```python
from build123d import *

# Parameters (mm, degrees)
SKETCH1_W           = 27
SKETCH1_H           = 24
BOSS_EXTRUDE1_DEPTH = 37
SHELL1_T            = -3.5
SKETCH3_R           = 2.1
CUT_EXTRUDE1_DEPTH  = 48.349762407
SKETCH5_W           = 74
SKETCH5_H           = 0.5
CUT_EXTRUDE3_DEPTH  = 48.349762407
SWEEP1_START        = -13.5
SWEEP1_DEPTH        = 27
SWEEP1_2_DEPTH      = 3.5
SWEEP1_START_2      = 10
SWEEP1_3_DEPTH      = 3.5


# Read off the part's stored shape, not the designer's step: Sweep1
with BuildPart() as part:
    # Sketch1 → Boss-Extrude1 (new, symmetric)
    with BuildSketch(Plane.XY):
        Rectangle(SKETCH1_W, SKETCH1_H)
    extrude(amount=BOSS_EXTRUDE1_DEPTH, both=True)

    # Shell1
    shell1_openings = [part.faces().sort_by_distance(p)[0] for p in [
        (0, 0, 37),
        (0, 0, -37),
        (0, -12, 0),
    ]]
    offset(amount=SHELL1_T, openings=shell1_openings, kind=Kind.INTERSECTION)

    # Sketch3 → Cut-Extrude1 (cut, through all)
    with BuildSketch(Plane.ZY.offset(13.5)):
        with Locations((-30, -1.5)):
            Circle(SKETCH3_R)
        with Locations((-10, -1.5)):
            Circle(SKETCH3_R)
        with Locations((10, -1.5)):
            Circle(SKETCH3_R)
        with Locations((30, -1.5)):
            Circle(SKETCH3_R)
    extrude(amount=-CUT_EXTRUDE1_DEPTH, mode=Mode.SUBTRACT)

    # Sketch5 → Cut-Extrude3 (cut, through all)
    with BuildSketch(Plane.ZY.offset(13.5)):
        with Locations((0, -11.75)):
            Rectangle(SKETCH5_W, SKETCH5_H)
    extrude(amount=-CUT_EXTRUDE3_DEPTH, mode=Mode.SUBTRACT)

    # Sweep1 outline → Sweep1 (add)
    with BuildSketch(Plane.YZ.offset(SWEEP1_START)):
        with BuildLine():
            Line((14.288034431, 44.256718109), (59.173181861, 108.359351944))
            Line((59.173181861, 108.359351944), (56.306149706, 110.366869471))
            Line((56.306149706, 110.366869471), (11.421002276, 46.264235636))
            ThreePointArc((11.421002276, 46.264235636), (9.247550016, 41.856910443), (8.5, 37))
            Line((8.5, 37), (12, 37))
            ThreePointArc((12, 37), (12.585559344, 40.804440145), (14.288034431, 44.256718109))
        make_face()
    extrude(amount=SWEEP1_DEPTH)

    # Sweep1 2 outline → Sweep1 2 (add)
    with BuildSketch(Plane.YZ.offset(SWEEP1_START)):
        with BuildLine():
            Line((11.421002276, 46.264235636), (56.306149706, 110.366869471))
            Line((56.306149706, 110.366869471), (39.923108821, 121.838398198))
            Line((39.923108821, 121.838398198), (-4.96203861, 57.735764364))
            ThreePointArc((-4.96203861, 57.735764364), (-9.826788999, 47.871026434), (-11.5, 37))
            Line((-11.5, 37), (8.5, 37))
            ThreePointArc((8.5, 37), (9.247550016, 41.856910443), (11.421002276, 46.264235636))
        make_face()
    extrude(amount=SWEEP1_2_DEPTH)

    # Sweep1 3 outline → Sweep1 3 (add)
    with BuildSketch(Plane.YZ.offset(SWEEP1_START_2)):
        with BuildLine():
            Line((11.421002276, 46.264235636), (56.306149706, 110.366869471))
            Line((56.306149706, 110.366869471), (39.923108821, 121.838398198))
            Line((39.923108821, 121.838398198), (-4.96203861, 57.735764364))
            ThreePointArc((-4.96203861, 57.735764364), (-9.826788999, 47.871026434), (-11.5, 37))
            Line((-11.5, 37), (8.5, 37))
            ThreePointArc((8.5, 37), (9.247550016, 41.856910443), (11.421002276, 46.264235636))
        make_face()
    extrude(amount=SWEEP1_3_DEPTH)


solid = part.part
```
Can you work these out from the model? Positions are in its coordinate system, mm. A direction names the side the tool comes from. Give positions to 0.01 mm unless a question says otherwise; leave off trailing zeros. Order: outer loops, then holes, each group sorted by start corner. A loop starts at its lowest first (then second) coordinate and runs counter-clockwise, first axis right, second up. Notation, with made-up numbers: M 13.25,-13.5 L 19.25,-13.5 A20 cw 19.25,19.5 Z; hole C 29.5,63 d4. An arc over 180 degrees is marked long. Write item = value, one per line. Start each with the question number.
Q1. Suppose I cut it at C-C (y = 5). Write out the boundary of the cut face in (x, z).
Q2. I need wall thicknesses on probe 1 along X at (y, z) = (3.5, 56); probe 2 along Y at (x, z) = (-12.6, 30); probe 3 along Y at (x, z) = (5, 31). Which ranges of each line are inside material? Lowest first, please. Write a range as [from, to].
Q3. We'd pull the mould along Z, two halves only. Please class faces 1 (the cylindrical face through (-11.77, -9.78, 48.02)), 2 (the flat face through (10, 7, 43)), 3 (the cylindrical face through (11.73, -1.41, 7.9)): pulls with the +Z half, pulls with the -Z half, needs draft (parallel to the pull), parting line crosses it, or undercut.
Q4. Will these pins go through, and if not, where does the flat tip stop? pin 1 Ø1.5 at (x, z) = (-6, 38.5) entering from -Y; pin 2 Ø3.5 at (y, z) = (-1.5, 30) entering from +X (1 decimal); pin 3 Ø8 at (x, z) = (3.5, 4.5) entering from +Y; pin 4 Ø6 at (x, y) = (-4.5, 34.5) entering from +Z.
Q5. Suppose I cut it at A-A (z = 30). Write out the boundary of the cut face in (x, y).
Q6. Suppose I cut it at B-B (x = 11.5). Write out the boundary of the cut face in (y, z), plus the area to 3 significant figures.
Q7. Suppose I cut it at D-D (z = 2.5). Write out the boundary of the cut face in (x, y).
Q8. For faces 4 (the cylindrical face through (11.73, -1.41, 27.9)), 5 (the cylindrical face through (-0.14, 9.268, 41.923)), 6 (the flat face through (0, 12, 1)), which set-ups out of +Z, -Z, +X, -X, +Y, -Y let a thin tool reach every point of the face, with its end or its side?
Check result:
q1.outline = M -13.5,-37 L -10,-37 L -10,71.96 L -13.5,71.96 Z; M 10,-37 L 13.5,-37 L 13.5,71.96 L 10,71.96 Z
q2.probe_1 = [-13.5, -10], [10, 13.5]
q2.probe_2 = [-11.5, -3.6], [0.6, 12]
q2.probe_3 = [8.5, 12]
q3.face_1 = pulls with the +Z half
q3.face_2 = needs draft
q3.face_3 = undercut
q4.pin_1 = 8.52
q4.pin_2 = through
q4.pin_3 = 12
q4.pin_4 = 83.51
q5.outline = M -13.5,-11.5 L -10,-11.5 L -10,-3.6 L -13.5,-3.6 Z; M -13.5,0.6 L -10,0.6 L -10,8.5 L 10,8.5 L 10,0.6 L 13.5,0.6 L 13.5,12 L -13.5,12 Z; M 10,-11.5 L 13.5,-11.5 L 13.5,-3.6 L 10,-3.6 Z
q6.outline = M -11.5,-37 L 12,-37 L 12,37 A12.65 cw 14.29,44.26 L 59.17,108.36 L 39.92,121.84 L -4.96,57.74 A36.15 ccw -11.5,37 Z; hole C -1.5,-30 d4.2; hole C -1.5,-10 d4.2; hole C -1.5,10 d4.2; hole C -1.5,30 d4.2
q6.area = 3,870 mm2
q7.outline = M -13.5,-11.5 L -10,-11.5 L -10,8.5 L 10,8.5 L 10,-11.5 L 13.5,-11.5 L 13.5,12 L -13.5,12 Z
q8.face_4 = +X, -X
q8.face_5 = +Z, -Y
q8.face_6 = -Z, +X, -X, +Y
